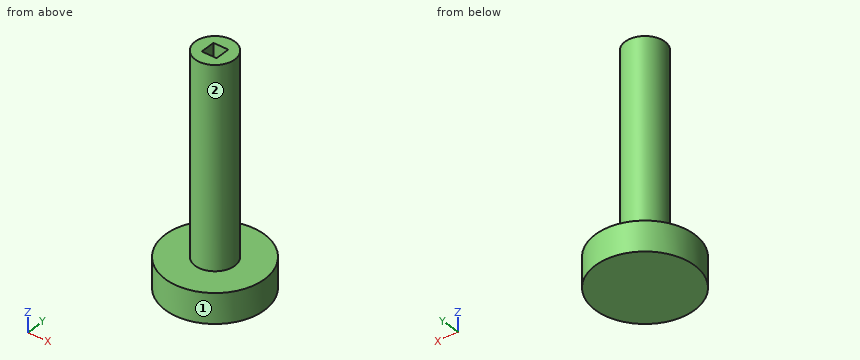
from build123d import *

# Parameters (mm, degrees)
F0_R     = 10
F1_DEPTH = 6
F2_R     = 4
F3_DEPTH = 40
F4_W     = 3
F4_H     = 3
F5_DEPTH = 5


with BuildPart() as f1:
    # F0 (on Top) → F1 (new body)
    with BuildSketch(Plane.XY):
        Circle(F0_R)
    extrude(amount=F1_DEPTH)

    # F2 (on face) → F3 (join)
    with BuildSketch(Plane.XY.offset(6)):
        Circle(F2_R)
    extrude(amount=F3_DEPTH)

    # F4 (on face) → F5 (cut)
    with BuildSketch(Plane.XY.offset(46)):
        Rectangle(F4_W, F4_H)
    extrude(amount=-F5_DEPTH, mode=Mode.SUBTRACT)


solid = f1.part
Part model, mm, in its own coordinate system. Face numbers are marked on the shaded views. A direction names the side the tool comes from. Coordinates: 2 decimals unless noted, no trailing zeros. Order: outer loops, then holes, each group sorted by start corner. A loop starts at its lowest first (then second) coordinate and runs counter-clockwise, first axis right, second up. Notation, with made-up numbers: M 30.5,34 L 74.5,34 A12 cw 74.5,48 Z; hole C -4.5,56.25 d10. An arc over 180 degrees is marked long. One line per question, with ' | ' between items.
Q1. Pin check, flat tips, straight feed: P1, Ø0.9, axis at x = 0.5, y = -0.5, coming from the +Z side; P2, Ø3.5, axis at y = -0.5, z = 44.5, coming from the +X side; P3, Ø3.5, axis at x = -0.5, z = 44, coming from the -Y side; P4, Ø2, axis at x = 6.5, z = 28, coming from the -Y side. Stop position of each tip, or through.
A:
P1: stops at z = 41 | P2: stops at x = 4 | P3: stops at y = -4 | P4: passes through
Q2. Slice it at D-D (z = 10). Give the cut face in (x, y).
A:
outline: C 0,0 d8
Q3. Slice it at B-B (z = 42). Give the cut face in (x, y), and give its area (3 significant figures).
A:
outline: C 0,0 d8; hole M -1.5,-1.5 L 1.5,-1.5 L 1.5,1.5 L -1.5,1.5 Z | area: 41.3 mm^2
Q4. Slice it at A-A (y = 0). Give the cut face in (x, z).
A:
outline: M -10,0 L 10,0 L 10,6 L 4,6 L 4,46 L 1.5,46 L 1.5,41 L -1.5,41 L -1.5,46 L -4,46 L -4,6 L -10,6 Z
Q5. 3-axis set-ups, long thin cutter, end or side, ignore diameter. For the marked faces 1 and 2: which of +Z, -Z, +X, -X, +Y, -Y reach the whole face in a straight line?
A:
face 1: +Z, -Z | face 2: +Z
Q6. Drill centre lines: line 1 (Z direction, x = 7, y = -5); line 2 (Z direction, x = 0.5, y = 0.75); line 3 (Y direction, x = 0.25, z = 15.5). Where is each one in solid material? Low to high.
A:
line 1: z = 0 to 6 | line 2: z = 0 to 41 | line 3: y = -3.99 to 3.99
